Could you check a few things on this model? Use its own coordinates, in mm. A direction names the side the tool comes from. Coordinates: 2 decimals unless noted, no trailing zeros. Loops run counter-clockwise (first coordinate to the right, second up) from the corner with the lowest first, then second, coordinate; pieces in that order, holes last.
from build123d import *

# Parameters (mm, degrees)
SKETCH1_W           = 100
SKETCH1_H           = 89
BOSS_EXTRUDE1_DEPTH = 6
CHAMFER1_SIZE       = 6
SKETCH2_W           = 3
SKETCH2_H           = 89
CUT_EXTRUDE1_DEPTH  = 3
SKETCH4_R           = 1.75
CUT_EXTRUDE3_DEPTH  = 68.203050526


with BuildPart() as part:
    # Sketch1 → Boss-Extrude1 (new body)
    with BuildSketch(Plane.XY):
        Rectangle(SKETCH1_W, SKETCH1_H)
    extrude(amount=BOSS_EXTRUDE1_DEPTH)

    # Chamfer1
    chamfer1_edges = [part.edges().sort_by_distance(p)[0] for p in [
        (0, -44.5, 6),
        (0, 44.5, 6),
    ]]
    chamfer(chamfer1_edges, length=CHAMFER1_SIZE - 0.0001)  # a hair under: the kernel refuses the full size

    # Sketch2 → Cut-Extrude1 (cut)
    with BuildSketch(Plane.XY.offset(6)):
        with Locations((-44.5, 0)):
            Rectangle(SKETCH2_W, SKETCH2_H)
    extrude(amount=-CUT_EXTRUDE1_DEPTH, mode=Mode.SUBTRACT)

    # Sketch4 → Cut-Extrude3 (cut, through all)
    with BuildSketch(Plane(origin=(0, 0, 0), x_dir=(-1, 0, 0), z_dir=(0, 0, -1))):
        with Locations((0.5, 25)):
            Circle(SKETCH4_R)
        with Locations((0.5, -25)):
            Circle(SKETCH4_R)
    extrude(amount=-CUT_EXTRUDE3_DEPTH, mode=Mode.SUBTRACT)


solid = part.part
(1) Imagine slicing it at A-A, the plane x = -0.5. State how many separate pieces and enclosed holes the cut face has, and give its area (3 significant figures).
Answers:
separate pieces: 3
enclosed holes: 0
area: 456 mm2
(2) For pin 1 (3 mm diameter, centred on x = -0.5, y = -25, fed in from -Z); pin 2 (1 mm diameter, centred on x = -7.5, z = 3, fed in from -Y); pin 3 (1.5 mm diameter, centred on x = -45, y = 8, fed in from +Z); pin 4 (2 mm diameter, centred on x = 8, z = 5, fed in from -Y), each with a flat end and sliding along its axis, tell me the tip position at first contact or that it passes through.
Answers:
pin 1: passes through
pin 2: stops at y = -42
pin 3: stops at z = 3
pin 4: stops at y = -40.5
(3) Imagine slicing it at B-B, the plane y = -25. Write out the boundary of the cut face in (x, z).
Answers:
outline: (-50, 0) - (-2.25, 0) - (-2.25, 6) - (-43, 6) - (-43, 3) - (-46, 3) - (-46, 6) - (-50, 6) - close; (1.25, 0) - (50, 0) - (50, 6) - (1.25, 6) - close
(4) I need wall thicknesses on probe 1 along X at (y, z) = (21, 5.75); probe 2 along Y at (x, z) = (-0.5, 4.5); probe 3 along Y at (x, z) = (-0.5, 4.7). Which ranges of each line are inside material? Lowest first, please.
Answers:
probe 1: x = -50 to -46, -43 to 50
probe 2: y = -40 to -26.75, -23.25 to 23.25, 26.75 to 40
probe 3: y = -39.8 to -26.75, -23.25 to 23.25, 26.75 to 39.8
(5) Which directions (+Z, -Z, +X, -X, +Y, -Y) give clear straight access to the entire face, cutting with the end or side of a thin tool? Please do faces 4 (the face through (50, -1, 3)), 5 (the face through (-43, -1, 5)).
Answers:
face 4: +Z, -Z, +X, +Y, -Y
face 5: +Z, +Y, -Y
(6) We'd pull the mould along Y, two halves only. Please class faces 1 (the face through (-0.272, -23.265, 2.958)), 2 (the face through (-48, 1, 6)), 3 (the face through (-0.7, 41.5, 3)): +Y half, -Y half, draft (parallel to the pull), parting line (faces both ways), or undercut.
Answers:
face 1: undercut
face 2: draft
face 3: +Y half
(7) Imagine slicing it at C-C, the plane y = -16. Write out the boundary of the cut face in (x, z).
Answers:
outline: (-50, 0) - (50, 0) - (50, 6) - (-43, 6) - (-43, 3) - (-46, 3) - (-46, 6) - (-50, 6) - close
